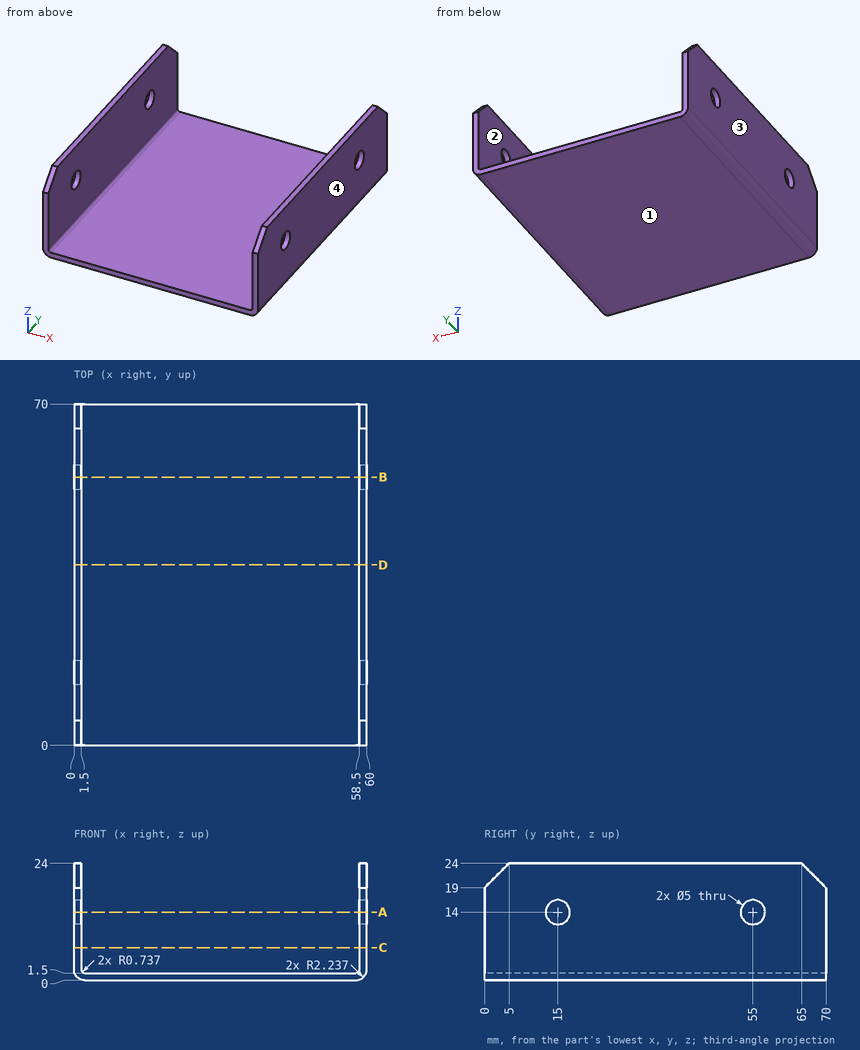
Part print with two shaded views. Sizes in mm from the minimum x, y, z corner. Coordinates: 2 decimals unless noted, no trailing zeros. Loops run counter-clockwise (first coordinate to the right, second up) from the corner with the lowest first, then second, coordinate; pieces in that order, holes last. Notation, with made-up numbers: (73, 69.25) -> (84, 69.25) arc R16 cw to (84, 90.25) -> close; hole circle Ø3 at (1.25, 35.5). An arc over 180 degrees is marked (long way). Answer as a JSON object with one key per item and string values.
Q1. Cut at B-B (y = 55). List the corners of the cut face in (x, z).
Report:
{"outline": "(0, 2.24) arc R2.24 ccw to (2.24, 0) -> (57.76, 0) arc R2.24 ccw to (60, 2.24) -> (60, 11.5) -> (58.5, 11.5) -> (58.5, 2.24) arc R0.74 cw to (57.76, 1.5) -> (2.24, 1.5) arc R0.74 cw to (1.5, 2.24) -> (1.5, 11.5) -> (0, 11.5) -> close; (0, 16.5) -> (1.5, 16.5) -> (1.5, 24) -> (0, 24) -> close; (58.5, 16.5) -> (60, 16.5) -> (60, 24) -> (58.5, 24) -> close"}
Q2. Cut at D-D (y = 37). List the corners of the cut face in (x, z).
Report:
{"outline": "(0, 2.24) arc R2.24 ccw to (2.24, 0) -> (57.76, 0) arc R2.24 ccw to (60, 2.24) -> (60, 24) -> (58.5, 24) -> (58.5, 2.24) arc R0.74 cw to (57.76, 1.5) -> (2.24, 1.5) arc R0.74 cw to (1.5, 2.24) -> (1.5, 24) -> (0, 24) -> close"}
Q3. Cut at C-C (z = 6.75). List the corners of the cut face in (x, y), and give its area (3 significant figures).
Report:
{"outline": "(0, 0) -> (1.5, 0) -> (1.5, 70) -> (0, 70) -> close; (58.5, 0) -> (60, 0) -> (60, 70) -> (58.5, 70) -> close", "area": "210 mm2"}
Q4. Flat gauge pins, fed straight in: P1, Ø16.5, axis at x = 23, y = 42.5, coming from the +Z side; P2, Ø6.5, axis at y = 55, z = 14, coming from the +X side; P3, Ø4, axis at y = 55, z = 14, coming from the +X side. Where does each tip first touch, or does it go through?
Report:
{"P1": "stops at z = 1.5", "P2": "stops at x = 60", "P3": "passes through"}
Q5. Cut at A-A (z = 14). List the corners of the cut face in (x, y), and give its area (3 significant figures).
Report:
{"outline": "(0, 0) -> (1.5, 0) -> (1.5, 12.5) -> (0, 12.5) -> close; (0, 17.5) -> (1.5, 17.5) -> (1.5, 52.5) -> (0, 52.5) -> close; (0, 57.5) -> (1.5, 57.5) -> (1.5, 70) -> (0, 70) -> close; (58.5, 0) -> (60, 0) -> (60, 12.5) -> (58.5, 12.5) -> close; (58.5, 17.5) -> (60, 17.5) -> (60, 52.5) -> (58.5, 52.5) -> close; (58.5, 57.5) -> (60, 57.5) -> (60, 70) -> (58.5, 70) -> close", "area": "180 mm2"}
Q6. Pull direction X, two halves, no side cores. Call the marked faces 1, 2, 3 and 4: released by +X, released by -X, zero draft, split by the parting line, or undercut.
Report:
{"face 1": "zero draft", "face 2": "undercut", "face 3": "released by -X", "face 4": "released by +X"}
Q7. Probe probe 1 along Y at (x, z) = (1.2, 14); probe 2 along X at (y, z) = (48, 23); probe 3 along Z at (x, y) = (6, 18). List the from-to ranges inside material, lowest first.
Report:
{"probe 1": "y = 0 to 12.5, 17.5 to 52.5, 57.5 to 70", "probe 2": "x = 0 to 1.5, 58.5 to 60", "probe 3": "z = 0 to 1.5"}
